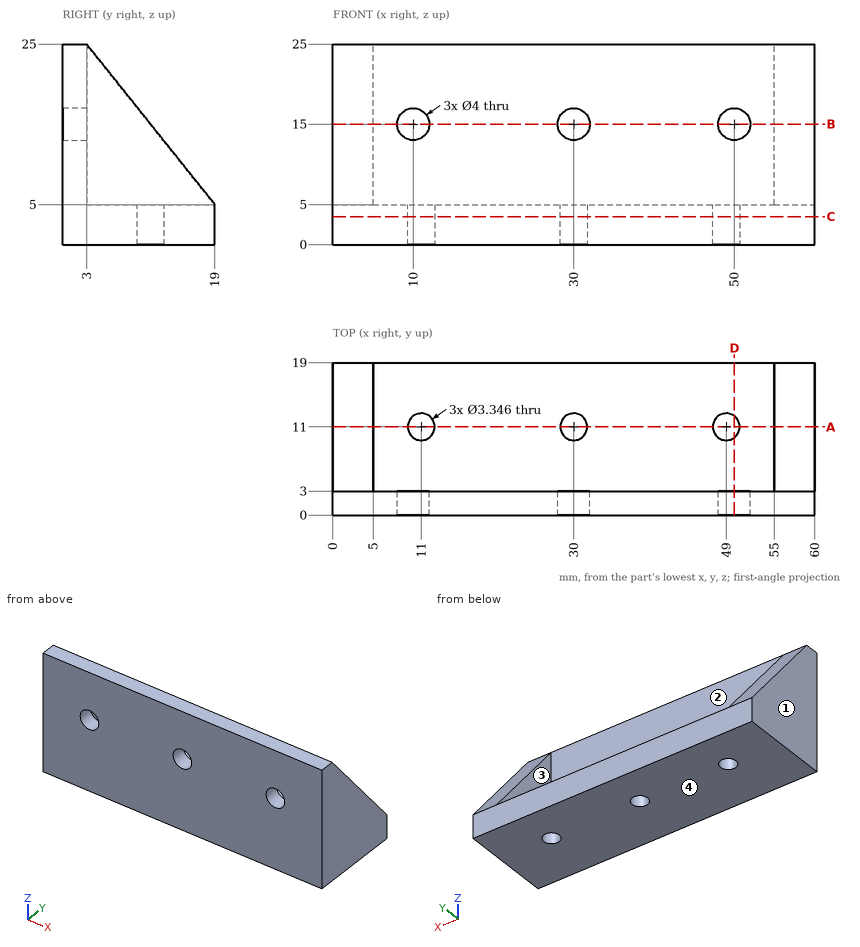
The drawing under review shows one solid part. Ordinate dimensions are in mm from its lowest x, y, z. Round coordinates to 2 decimals unless told otherwise and drop trailing zeros. Write each loop counter-clockwise with the first axis right and the second up, starting at its lowest first coordinate (ties: lowest second). Pieces come first, ordered by that corner, then holes.
(1) We need section D-D on x = 50. Give the boundary of the cut face in (y, z), and give its area (3 significant figures).
(2) We need section A-A on y = 11. Give the boundary of the cut face in (x, z).
(3) We need section C-C on z = 3.5. Give the boundary of the cut face in (x, y), and give its area (3 significant figures).
(4) Wall thickness on L1, parallel to X at y = 1.7, z = 15; L2, parallel to X at y = 3.75, z = 7.5; L3, parallel to X at y = 2, z = 16.25: over which ranges is each line inside the solid? List them lowest first.
(5) Mouldability with a two-part tool opening along X and no side actions: class the marked faces 1, 2, 3 and 4 as +X half, -X half, draft (parallel to the pull), parting line (faces both ways), or undercut.
(6) Insertion check: pin 1 (4 mm diameter, centred on x = 20, z = 17.5, fed in from -Y); pin 2 (4.5 mm diameter, centred on x = 50, z = 15, fed in from +Y); pin 3 (3 mm diameter, centred on x = 30, z = 15, fed in from +Y); pin 4 (4 mm diameter, centred on x = 49, y = 11, fed in from +Z). Each pin has a flat end and moves straight along its axis. Give the tip position at first contact, or say it passes through.
(7) We need section B-B on z = 15. Give the boundary of the cut face in (x, y), and give its area (3 significant figures).
Findings below:
1. outline: (0, 0) - (9.66, 0) - (9.66, 5) - (3, 5) - (3, 13) - (0, 13) - close; (0, 17) - (3, 17) - (3, 25) - (0, 25) - close; (12.34, 0) - (19, 0) - (19, 5) - (12.34, 5) - close
1. area: 130 mm2
2. outline: (0, 0) - (9.33, 0) - (9.33, 5) - (5, 5) - (5, 15) - (0, 15) - close; (12.67, 0) - (28.33, 0) - (28.33, 5) - (12.67, 5) - close; (31.67, 0) - (47.33, 0) - (47.33, 5) - (31.67, 5) - close; (50.67, 0) - (60, 0) - (60, 15) - (55, 15) - (55, 5) - (50.67, 5) - close
3. outline: (0, 0) - (60, 0) - (60, 19) - (0, 19) - close; hole circle Ø3.35 at (11, 11); hole circle Ø3.35 at (30, 11); hole circle Ø3.35 at (49, 11)
3. area: 1,110 mm2
4. L1: x = 0 to 8, 12 to 28, 32 to 48, 52 to 60
4. L2: x = 0 to 5, 55 to 60
4. L3: x = 0 to 8.44, 11.56 to 28.44, 31.56 to 48.44, 51.56 to 60
5. face 1: -X half
5. face 2: undercut
5. face 3: undercut
5. face 4: draft
6. pin 1: stops at y = 0
6. pin 2: stops at y = 3
6. pin 3: passes through
6. pin 4: stops at z = 5
7. outline: (0, 0) - (8, 0) - (8, 3) - (5, 3) - (5, 11) - (0, 11) - close; (12, 0) - (28, 0) - (28, 3) - (12, 3) - close; (32, 0) - (48, 0) - (48, 3) - (32, 3) - close; (52, 0) - (60, 0) - (60, 11) - (55, 11) - (55, 3) - (52, 3) - close
7. area: 224 mm2
